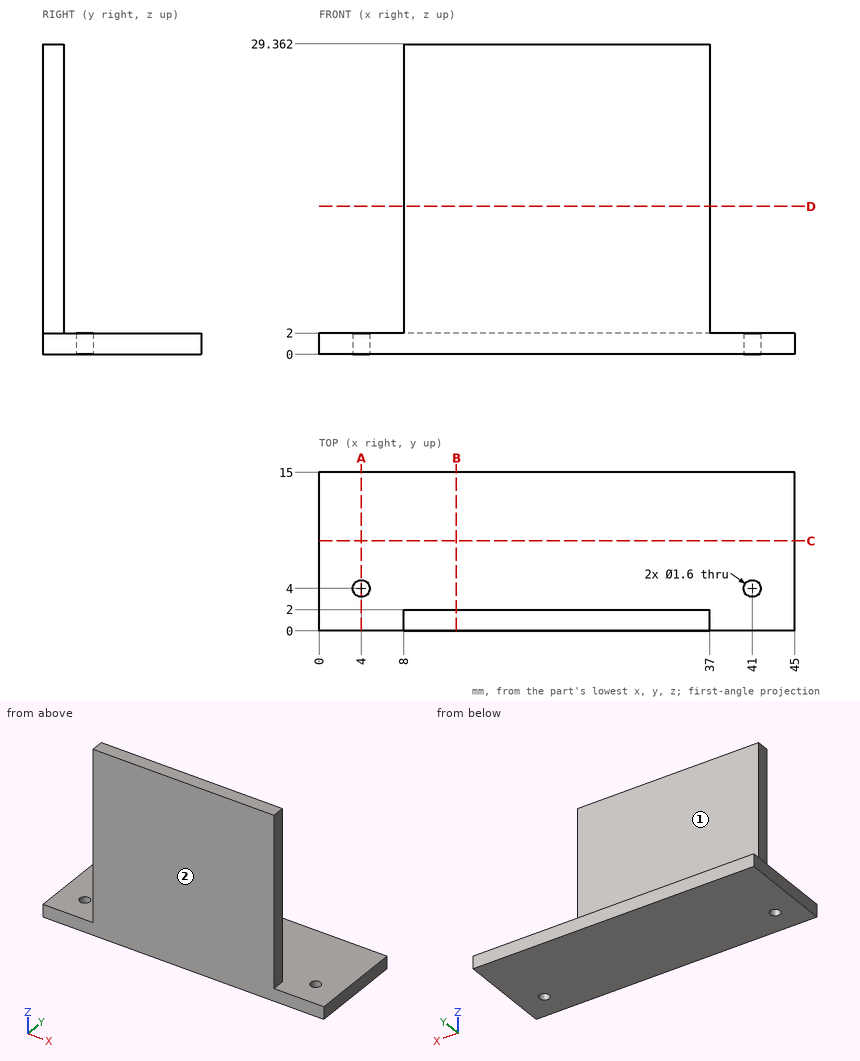
Study the drawing (mm; zero at the part's minimum x, y, z) and answer. A direction names the side the tool comes from. Coordinates: 2 decimals unless noted, no trailing zeros. Write each loop counter-clockwise with the first axis right and the second up, starting at its lowest first coordinate (ties: lowest second). Pieces come first, ordered by that corner, then holes. Notation, with made-up numbers: (-1.75, -2.75) -> (57.25, -2.75) arc R28 cw to (57.25, 28.25) -> close; hole circle Ø6 at (75, 58). An arc over 180 degrees is marked (long way). Write each question's results on one line, items separated by ' | '. Start each with the question number.
1) A cutting plane is placed at B-B (x = 13). Determine the outline of the cut face in (y, z).
2) Flat-ended cylindrical pins translate along their axes: pin 1 Ø1.6 at (y, z) = (1, 17) entering from +X; pin 2 Ø2 at (x, y) = (4, 4) entering from +Z; pin 3 Ø0.6 at (y, z) = (0.5, 18.5) entering from -X; pin 4 Ø4 at (y, z) = (5.5, 25) entering from -X. Find the tip coordinate at first contact, or state that the pin passes through.
3) A cutting plane is placed at C-C (y = 8.5). Determine the outline of the cut face in (x, z).
4) A cutting plane is placed at A-A (x = 4). Determine the outline of the cut face in (y, z), then the cut area to 3 significant figures.
5) A tool of negligible diameter and unlimited length cuts with its end or side. For the marked faces 1 and 2, from which of +Z, -Z, +X, -X, +Y, -Y can it reach the whole face along a straight path? Write none if from no direction.
6) Straight lines are drawn through the part: probe 1 along Y at (x, z) = (41, 1.1); probe 2 along Y at (x, z) = (28, 17.25). For each, find the intervals that lie inside material, in ascending order.
7) A cutting plane is placed at D-D (z = 14). Determine the outline of the cut face in (x, y).
Values follow:
1) outline: (0, 0) -> (15, 0) -> (15, 2) -> (2, 2) -> (2, 29.36) -> (0, 29.36) -> close
2) pin 1: x = 37 | pin 2: z = 2 | pin 3: x = 8 | pin 4: through
3) outline: (0, 0) -> (45, 0) -> (45, 2) -> (0, 2) -> close
4) outline: (0, 0) -> (3.2, 0) -> (3.2, 2) -> (0, 2) -> close; (4.8, 0) -> (15, 0) -> (15, 2) -> (4.8, 2) -> close | area: 26.8 mm²
5) face 1: +Z, +X, -X, +Y | face 2: +Z, -Z, +X, -X, -Y
6) probe 1: 0 to 3.2, 4.8 to 15 | probe 2: 0 to 2
7) outline: (8, 0) -> (37, 0) -> (37, 2) -> (8, 2) -> close
